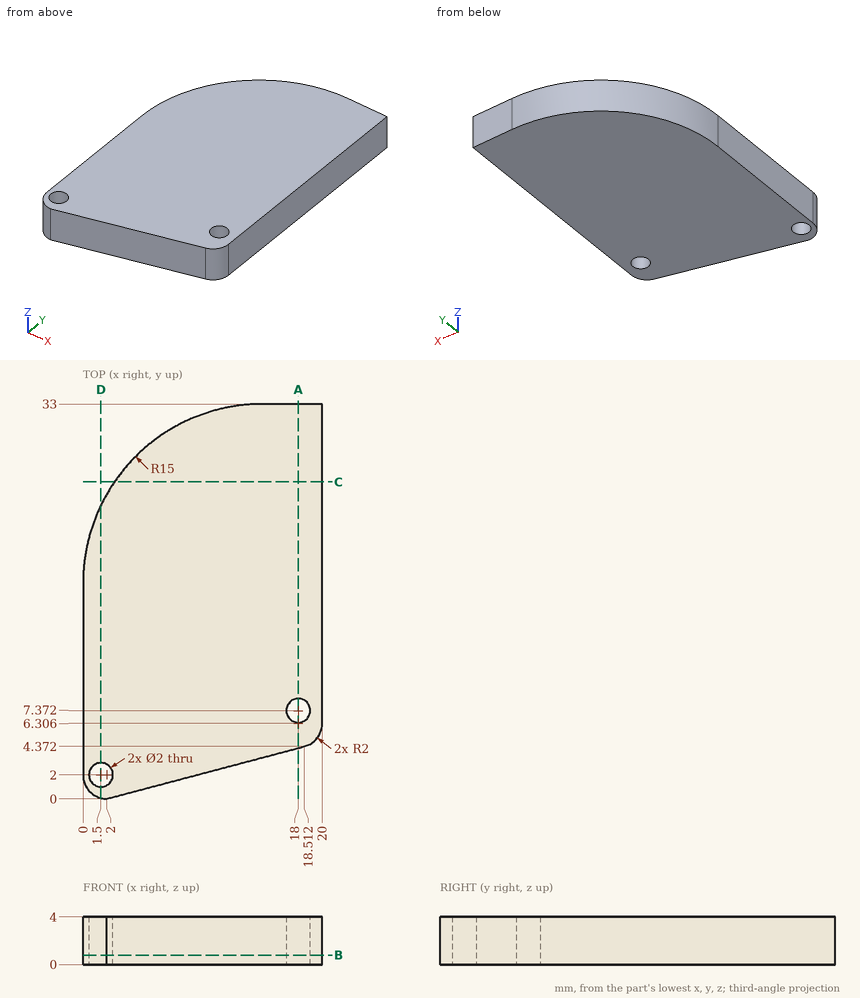
Design review of the part shown in the three views and the two pictorial views. Dimensions are in mm from the part's minimum x, y and z. Give positions to 0.01 mm unless a question says otherwise; leave off trailing zeros. Write each loop counter-clockwise with the first axis right and the second up, starting at its lowest first coordinate (ties: lowest second). Pieces come first, ordered by that corner, then holes. Notation, with made-up numbers: (-19.75, 0.5) -> (38.25, 0.5) arc R20 ccw to (38.25, 21.5) -> close; hole circle Ø8 at (83, 12.5). An arc over 180 degrees is marked (long way). Answer in a Markdown table with one row per item.
1) Add section D-D on x = 1.5. State the section outline as (y, z) points.
Worked answers:
| item | result |
|---|---|
| outline | (0.06, 0) -> (1, 0) -> (1, 4) -> (0.06, 4) -> close; (3, 0) -> (24.54, 0) -> (24.54, 4) -> (3, 4) -> close |
2) Add section C-C on y = 26.5. State the section outline as (x, z) points.
Worked answers:
| item | result |
|---|---|
| outline | (2.64, 0) -> (20, 0) -> (20, 4) -> (2.64, 4) -> close |
3) Add section B-B on z = 0.8. State the section outline as (x, y) points (1 decimal).
Worked answers:
| item | result |
|---|---|
| outline | (0, 2) arc R2 ccw to (2, 0) -> (18.5, 4.4) arc R2 ccw to (20, 6.3) -> (20, 33) -> (15, 33) arc R15 ccw to (0, 18) -> close; hole circle Ø2 at (1.5, 2); hole circle Ø2 at (18, 7.4) |
4) Add section A-A on x = 18. State the section outline as (y, z) points, plus the area to 3 significant figures.
Worked answers:
| item | result |
|---|---|
| outline | (4.24, 0) -> (6.37, 0) -> (6.37, 4) -> (4.24, 4) -> close; (8.37, 0) -> (33, 0) -> (33, 4) -> (8.37, 4) -> close |
| area | 107 mm² |
5) For L1, parallel to X at y = 8, z = 3.2; L2, parallel to Y at x = 1.5, z = 1.6 (1 decimal); L3, parallel to X at y = 5, z = 0.5 (1 decimal), list the stretches that pass through material, from the lowest coordinate up. Write a range as [from, to].
Worked answers:
| item | result |
|---|---|
| L1 | [0, 17.22], [18.78, 20] |
| L2 | [0.1, 1], [3, 24.5] |
| L3 | [0, 19.5] |
6) Clearance check with a flat-ended pin moving along its axis: P1, Ø1.2, axis at x = 1.5, y = 2, coming from the +Z side. State where the tip first meets the part, or that it passes through.
Worked answers:
| item | result |
|---|---|
| P1 | through |
